Verification items for the finished model (mm, model axes). Round coordinates to 2 decimals unless told otherwise and drop trailing zeros. Order: outer loops, then holes, each group sorted by start corner. A loop starts at its lowest first (then second) coordinate and runs counter-clockwise, first axis right, second up. Notation, with made-up numbers: M 79.5,-24 L 104.5,-24 A3 ccw 104.5,-20 Z; hole C -29,1.5 d3. An arc over 180 degrees is marked long. Use one line per item in the form item = value. Start each with the question number.
Item 1: Cross-section at C-C on x = 66.5. Enter the section's corners in (y, z), then the cut area to 3 significant figures.
Item 2: Release check for a two-part mould opening along X. For faces 1 (the flat face through (240, 19, -2)), 2 (the flat face through (128, -20, -4)), 3 (the cylindrical face through (31.776, -35.139, -1.972)) record: +X half, -X half, draft (parallel to the pull), parting line (faces both ways), or undercut.
Item 3: Go/stop test with flat-tipped pins: pin 1 Ø12 at (x, y) = (59.5, 20.5) entering from -Z; pin 2 Ø2 at (x, z) = (231, -2.5) entering from -Y; pin 3 Ø0.6 at (x, z) = (209.5, -2) entering from -Y; pin 4 Ø2 at (y, z) = (-56.5, -1.5) entering from +X. Record where each tip stops, or that it passes through.
Item 4: Cross-section at A-A on x = 130. Enter the section's corners in (y, z).
Item 5: Cross-section at B-B on x = 192. Enter the section's corners in (y, z).
Item 6: Thickness scan on probe 1 along Y at (x, z) = (101, -3.65); probe 2 along Y at (x, z) = (144, -2.6); probe 3 along X at (y, z) = (-44, -2.1). Record the ranges inside material, lowest first. Write a range as [from, to].
from build123d import *

# Parameters (mm, degrees)
SKETCH_1_R             = 9.5
SKETCH_1_R_2           = 1.5
SKETCH_1_W             = 20.5
SKETCH_1_H             = 4.1
SM_BASE_FLANGE_1_DEPTH = 4
SKETCH_6_R             = 1.75
CUT_EXTRUDE_1_DEPTH    = 267.640207021
SKETCH_8_R             = 1
SKETCH_8_R_2           = 0.822154456
CUT_EXTRUDE_3_DEPTH    = 10
CUT_EXTRUDE_4_REACH    = 268.64
SKETCH_9_R             = 1.5


# Sheet-metal steps are written as plain solids
with BuildPart() as part:
    # Sketch 1 → Базовая кромка1 (new body)
    with BuildSketch(Plane.XY):
        with BuildLine():
            Line((52, -59), (60, -59))
            Line((60, -59), (60, -55))
            Line((60, -55), (200, -55))
            Line((200, -55), (200, -59))
            Line((200, -59), (208, -59))
            Line((208, -59), (208, -55))
            Line((208, -55), (206, -55))
            Line((206, -55), (206, -51))
            Line((206, -51), (214, -51))
            Line((214, -51), (214, -55))
            Line((214, -55), (212, -55))
            Line((212, -55), (212, -59))
            Line((212, -59), (220, -59))
            Line((220, -59), (220, -55))
            Line((220, -55), (260, -55))
            Line((260, -55), (260, -1))
            Line((260, -1), (220, 39))
            Line((220, 39), (120, 39))
            Line((120, 39), (114, 39))
            ThreePointArc((114, 39), (111.171572875, 37.828427125), (110, 35))
            Line((110, 35), (110, 15))
            ThreePointArc((110, 15), (108.828427125, 12.171572875), (106, 11))
            Line((106, 11), (4, 11))
            ThreePointArc((4, 11), (1.171572875, 9.828427125), (0, 7))
            Line((0, 7), (0, 0))
            Line((0, 0), (0, -55))
            Line((0, -55), (40, -55))
            Line((40, -55), (40, -59))
            Line((40, -59), (48, -59))
            Line((48, -59), (48, -55))
            Line((48, -55), (46, -55))
            Line((46, -55), (46, -51))
            Line((46, -51), (54, -51))
            Line((54, -51), (54, -55))
            Line((54, -55), (52, -55))
            Line((52, -55), (52, -59))
        make_face()
        with Locations((23, -31.5)):
            Circle(SKETCH_1_R, mode=Mode.SUBTRACT)
        with Locations((156, -43)):
            Circle(SKETCH_1_R_2, mode=Mode.SUBTRACT)
        with Locations((206.7, 0.4)):
            Circle(SKETCH_1_R_2, mode=Mode.SUBTRACT)
        with Locations((156, 0.4)):
            Circle(SKETCH_1_R_2, mode=Mode.SUBTRACT)
        with Locations((206.7, -44.2)):
            Circle(SKETCH_1_R_2, mode=Mode.SUBTRACT)
        with Locations((144, -47)):
            Circle(SKETCH_1_R_2, mode=Mode.SUBTRACT)
        with Locations((216, -47)):
            Circle(SKETCH_1_R_2, mode=Mode.SUBTRACT)
        with Locations((216, 13)):
            Circle(SKETCH_1_R_2, mode=Mode.SUBTRACT)
        with Locations((144, 13)):
            Circle(SKETCH_1_R_2, mode=Mode.SUBTRACT)
        with Locations((30, -6.05)):
            Rectangle(SKETCH_1_W, SKETCH_1_H, mode=Mode.SUBTRACT)
        with Locations((230, -6.169027082)):
            Rectangle(SKETCH_1_W, SKETCH_1_H, mode=Mode.SUBTRACT)
        with Locations((126, -6.05)):
            Rectangle(SKETCH_1_W, SKETCH_1_H, mode=Mode.SUBTRACT)
    extrude(amount=-SM_BASE_FLANGE_1_DEPTH)

    # Эскиз6 → Вырез-Вытянуть1 (cut, through all)
    with BuildSketch(Plane.XY):
        with Locations((6, 5)):
            Circle(SKETCH_6_R)
        with Locations((120, 34)):
            Circle(SKETCH_6_R)
        with Locations((214, 34)):
            Circle(SKETCH_6_R)
        with Locations((245.514718626, 5)):
            Circle(SKETCH_6_R)
        with Locations((6, -14)):
            Circle(SKETCH_6_R)
        with Locations((6, -50)):
            Circle(SKETCH_6_R)
    extrude(amount=-CUT_EXTRUDE_1_DEPTH, mode=Mode.SUBTRACT)

    # Эскиз8 → Вырез-Вытянуть3 (cut)
    with BuildSketch(Plane.XZ.offset(55)):
        with Locations((210, -2)):
            Circle(SKETCH_8_R)
        with Locations((50, -2)):
            Circle(SKETCH_8_R_2)
    extrude(amount=-CUT_EXTRUDE_3_DEPTH, mode=Mode.SUBTRACT)

    # Эскиз9 → Вырез-Вытянуть4 (cut, up to next)
    with BuildSketch(Plane.XY, mode=Mode.PRIVATE) as cut_extrude_4_sk1:
        with Locations((60, -13.1)):
            Circle(SKETCH_9_R)
    cut_extrude_4_tool1 = extrude(cut_extrude_4_sk1.sketch, amount=-CUT_EXTRUDE_4_REACH, mode=Mode.PRIVATE) & part.part
    # Эскиз9 → Вырез-Вытянуть4 (cut, up to next)
    with BuildSketch(Plane.XY, mode=Mode.PRIVATE) as cut_extrude_4_sk2:
        with Locations((101, -34.1)):
            Circle(SKETCH_9_R)
    cut_extrude_4_tool2 = extrude(cut_extrude_4_sk2.sketch, amount=-CUT_EXTRUDE_4_REACH, mode=Mode.PRIVATE) & part.part
    # Эскиз9 → Вырез-Вытянуть4 (cut, up to next)
    with BuildSketch(Plane.XY, mode=Mode.PRIVATE) as cut_extrude_4_sk3:
        with Locations((101, -13.1)):
            Circle(SKETCH_9_R)
    cut_extrude_4_tool3 = extrude(cut_extrude_4_sk3.sketch, amount=-CUT_EXTRUDE_4_REACH, mode=Mode.PRIVATE) & part.part
    # Эскиз9 → Вырез-Вытянуть4 (cut, up to next)
    with BuildSketch(Plane.XY, mode=Mode.PRIVATE) as cut_extrude_4_sk4:
        with Locations((60, -34.1)):
            Circle(SKETCH_9_R)
    cut_extrude_4_tool4 = extrude(cut_extrude_4_sk4.sketch, amount=-CUT_EXTRUDE_4_REACH, mode=Mode.PRIVATE) & part.part
    add(cut_extrude_4_tool1.solids().sort_by_distance((60, -13.1, 0))[0], mode=Mode.SUBTRACT)
    add(cut_extrude_4_tool2.solids().sort_by_distance((101, -34.1, 0))[0], mode=Mode.SUBTRACT)
    add(cut_extrude_4_tool3.solids().sort_by_distance((101, -13.1, 0))[0], mode=Mode.SUBTRACT)
    add(cut_extrude_4_tool4.solids().sort_by_distance((60, -34.1, 0))[0], mode=Mode.SUBTRACT)


solid = part.part
Output values:
q1.outline = M -55,-4 L 11,-4 L 11,0 L -55,0 Z
q1.area = 264 mm2
q2.face_1 = +X half
q2.face_2 = draft
q2.face_3 = undercut
q3.pin_1 = through
q3.pin_2 = -55
q3.pin_3 = -45
q3.pin_4 = 220
q4.outline = M -55,-4 L -8.1,-4 L -8.1,0 L -55,0 Z; M -4,-4 L 39,-4 L 39,0 L -4,0 Z
q5.outline = M -55,-4 L 39,-4 L 39,0 L -55,0 Z
q6.probe_1 = [-55, -35.6], [-32.6, -14.6], [-11.6, 11]
q6.probe_2 = [-55, -48.5], [-45.5, 11.5], [14.5, 39]
q6.probe_3 = [0, 154.88], [157.12, 205.21], [208.19, 260]
